Can you work these out from the model? Positions are in its coordinate system, mm. A direction names the side the tool comes from. Give positions to 0.01 mm unless a question says otherwise; leave off trailing zeros. Loops run counter-clockwise (first coordinate to the right, second up) from the corner with the lowest first, then second, coordinate; pieces in that order, holes last. Notation, with made-up numbers: (-24, -21) - (-15, -21) arc R15 cw to (-15, 4) - close; hole circle Ø2 at (-8, -1). An arc over 180 degrees is marked (long way). Write item = value, one per line.
from build123d import *

# Parameters (mm, degrees)
SKETCH1_R           = 9.525
BOSS_EXTRUDE1_DEPTH = 1.27
SKETCH2_R           = 8.3185
BOSS_EXTRUDE2_DEPTH = 10.541
SKETCH3_R           = 6.1722
CUT_EXTRUDE1_DEPTH  = 9.652
SKETCH4_R           = 1.27
CUT_EXTRUDE2_DEPTH  = 17.571431863


with BuildPart() as part:
    # Sketch1 → Boss-Extrude1 (new body)
    with BuildSketch(Plane.XY):
        Circle(SKETCH1_R)
    extrude(amount=BOSS_EXTRUDE1_DEPTH)

    # Sketch2 → Boss-Extrude2 (add)
    with BuildSketch(Plane(origin=(0, 0, 1.27), x_dir=(-1, 0, 0), z_dir=(0, 0, -1))):
        Circle(SKETCH2_R)
    extrude(amount=BOSS_EXTRUDE2_DEPTH)

    # Sketch3 → Cut-Extrude1 (cut)
    with BuildSketch(Plane.XY.offset(1.27)):
        Circle(SKETCH3_R)
    extrude(amount=-CUT_EXTRUDE1_DEPTH, mode=Mode.SUBTRACT)

    # Sketch4 → Cut-Extrude2 (cut, through all)
    with BuildSketch(Plane.XY.offset(-8.382)):
        with Locations((0, 3.937)):
            Circle(SKETCH4_R)
        with Locations(Location((0, -3.937, 0), (0, 0, 180))):
            Circle(SKETCH4_R)
    extrude(amount=-CUT_EXTRUDE2_DEPTH, mode=Mode.SUBTRACT)

    # Sketch5 → Cut-Revolve1 (revolve, cut)
    with BuildSketch(Plane(origin=(0, 0, 0), x_dir=(0, 0, -1), z_dir=(1, 0, 0))):
        Polygon((0, 7.1247), (0, 9.525), (9.271, 9.525), (9.271, 7.1247), (8.128, 7.1247), (8.128, 7.0485), (6.858, 7.0485), (6.858, 7.493), (5.08, 7.493), (5.08, 7.0485), (3.429, 7.0485), (3.429, 7.62), (1.651, 7.62), (1.651, 7.1247), align=None)
    revolve(axis=Axis((0, 0, 0), (0, 0, 1)), mode=Mode.SUBTRACT)


solid = part.part
Q1. I need wall thicknesses on L1, parallel to Z at x = 3, y = -6.5; L2, parallel to Y at x = 0, z = -8.7; L3, parallel to Y at x = 0, z = -2. Which ranges of each line are inside material? Lowest first, please.
Output:
L1 = -6.86 to -5.08, -3.43 to -1.65, 0 to 1.27
L2 = -7.12 to -5.21, -2.67 to 2.67, 5.21 to 7.12
L3 = -7.62 to -6.17, 6.17 to 7.62
Q2. Imagine slicing it at B-B, the plane z = -2.5. Write out the boundary of the cut face in (x, y), then the cut area to 3 significant figures.
Output:
outline = circle Ø15.24 at (0, 0); hole circle Ø12.34 at (0, 0)
area = 62.7 mm2
Q3. For pin 1 (5 mm diameter, centred on y = -5.5, z = -5.5, fed in from +X); pin 2 (6 mm diameter, centred on y = 0, z = -7.5, fed in from -X); pin 3 (3.5 mm diameter, centred on x = 0, y = 3.937, fed in from +Z), each with a flat end and sliding along its axis, tell me the tip position at first contact or that it passes through.
Output:
pin_1 = 6.87
pin_2 = -7.49
pin_3 = -8.38
Q4. Imagine slicing it at D-D, the plane x = 0. Give the number of separate pieces and of enclosed holes in the cut face, then the cut area to 3 significant figures.
Output:
separate_pieces = 3
enclosed_holes = 0
area = 35.3 mm2
Q5. Which directions (+Z, -Z, +X, -X, +Y, -Y) give clear straight access to the entire face, cutting with the end or side of a thin tool? Please do faces 4 (the cylindrical face through (-4.898, -3.756, -3.488)), 5 (the cylindrical face through (-4.815, -5.251, -0.814)), 6 (the cylindrical face through (-4.815, -5.251, -8.691)).
Output:
face_4 = +Z
face_5 = none
face_6 = -Z
Q6. We'd pull the mould along Y, two halves only. Please class faces 1 (the cylindrical face through (4.289, -5.593, -4.243)), 2 (the cylindrical face through (-0.586, -2.81, -8.82)), 3 (the flat face through (6.74, 2.79, -1.651)): released by +Y, released by -Y, zero draft, split by the parting line, or undercut.
Output:
face_1 = split by the parting line
face_2 = undercut
face_3 = zero draft
